Could you check a few things on this model? Use its own coordinates, in mm. Face numbers are marked on the shaded views. A direction names the side the tool comes from. Round coordinates to 2 decimals unless told otherwise and drop trailing zeros. Order: outer loops, then holes, each group sorted by start corner. A loop starts at its lowest first (then second) coordinate and runs counter-clockwise, first axis right, second up. Notation, with made-up numbers: (24.25, -19.5) -> (71.25, -19.5) arc R22 cw to (71.25, -9.5) -> close; hole circle Ø2 at (48, 9.25). An arc over 180 degrees is marked (long way). One line per question, with ' | ' between items.
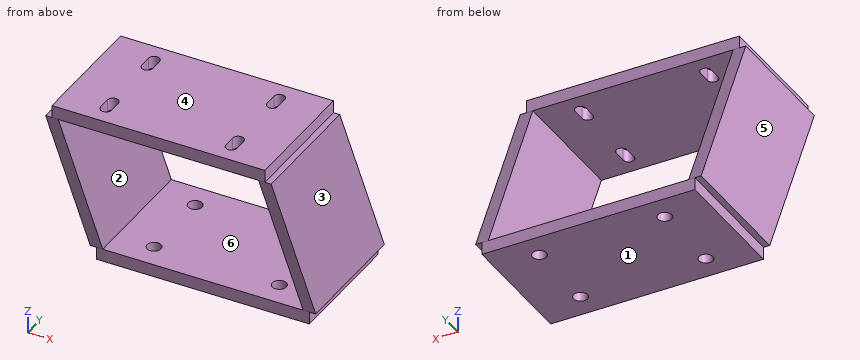
```python
from build123d import *

# Parameters (mm, degrees)
F0_W      = 215.9
F0_H      = 127
F1_DEPTH  = 12.7
F3_D      = 14.2875
F5_W      = 215.9
F5_H      = 127
F6_DEPTH  = 12.7
F8_DEPTH  = 212.726
F10_DEPTH = 6.35


# Not quite as in the source:
# - a length typed as a fraction of an inch, garbled in the dataset ("3 / 203.2 mm" for 3/8 in), is restored


with BuildPart() as f1:
    # F0 (on Top) → F1 (new body)
    with BuildSketch(Plane.XY):
        Rectangle(F0_W, F0_H)
    extrude(amount=F1_DEPTH)

    # F3 (through all)
    with Locations(Plane.XY.offset(12.7)):
        with Locations((-63.5, 38.1), (63.5, 38.1), (63.5, -38.1), (-63.5, -38.1)):
            Hole(F3_D / 2)



with BuildPart() as f6:
    # F5 (on offset) → F6 (new body)
    with BuildSketch(Plane.XY.offset(212.725)):
        with Locations((0, -82.55)):
            Rectangle(F5_W, F5_H)
    extrude(amount=-F6_DEPTH)

    # F7 (on face) → F8 (cut, through all)
    with BuildSketch(Plane.XY.offset(212.725)):
        with BuildLine():
            ThreePointArc((-57.94375, -38.1), (-63.5, -32.54375), (-69.05625, -38.1))
            Line((-69.05625, -38.1), (-69.05625, -50.8))
            ThreePointArc((-69.05625, -50.8), (-63.5, -56.35625), (-57.94375, -50.8))
            Line((-57.94375, -50.8), (-57.94375, -38.1))
        make_face()
        with BuildLine():
            ThreePointArc((-57.94375, -114.3), (-63.5, -108.74375), (-69.05625, -114.3))
            Line((-69.05625, -114.3), (-69.05625, -127))
            ThreePointArc((-69.05625, -127), (-63.5, -132.55625), (-57.94375, -127))
            Line((-57.94375, -127), (-57.94375, -114.3))
        make_face()
        with BuildLine():
            ThreePointArc((69.05625, -38.1), (63.5, -32.54375), (57.94375, -38.1))
            Line((57.94375, -38.1), (57.94375, -50.8))
            ThreePointArc((57.94375, -50.8), (63.5, -56.35625), (69.05625, -50.8))
            Line((69.05625, -50.8), (69.05625, -38.1))
        make_face()
        with BuildLine():
            ThreePointArc((69.05625, -114.3), (63.5, -108.74375), (57.94375, -114.3))
            Line((57.94375, -114.3), (57.94375, -127))
            ThreePointArc((57.94375, -127), (63.5, -132.55625), (69.05625, -127))
            Line((69.05625, -127), (69.05625, -114.3))
        make_face()
    extrude(amount=-F8_DEPTH, mode=Mode.SUBTRACT)


with BuildPart() as f1_1:
    add(f1.part)

    add(f6.part)  # F10 merges F6
    # F9 (on face) → F10 (join, symmetric)
    with BuildSketch(Plane.YZ.offset(107.95)):
        Polygon((63.5, 12.7), (-19.05, 200.025), (-146.05, 200.025), (-63.5, 12.7), align=None)
    extrude(amount=F10_DEPTH, both=True)

    # F11: F1 across plane


with BuildPart() as f1_2:
    add(f1_1.part)
    add(f1_1.part.mirror(Plane.YZ))


solid = f1_2.part
```
1. I want a section at A-A on x = 83. List the corners of the cut face in (y, z) for me (3 decimals), and give its area (3 significant figures).
From the geometry:
outline: (-146.05, 200.025) -> (-19.05, 200.025) -> (-19.05, 212.725) -> (-146.05, 212.725) -> close; (-63.5, 0) -> (63.5, 0) -> (63.5, 12.7) -> (-63.5, 12.7) -> close | area: 3,230 mm²
2. I want a section at D-D on y = -4.5. List the corners of the cut face in (x, z) for me, and give its area (3 significant figures).
From the geometry:
outline: (-114.3, 12.7) -> (-107.95, 12.7) -> (-107.95, 0) -> (107.95, 0) -> (107.95, 12.7) -> (114.3, 12.7) -> (114.3, 167.01) -> (101.6, 167.01) -> (101.6, 12.7) -> (-101.6, 12.7) -> (-101.6, 167.01) -> (-114.3, 167.01) -> close | area: 6,660 mm²
3. On a 3-axis mill with a long thin cutter (end or side, diameter ignored), from which of +Z, -Z, +X, -X, +Y, -Y can I reach the whole of each face in a straight line? I mean the marked faces 1 and 2. Say none if no direction works.
From the geometry:
face 1: -Z, +X, -X, +Y, -Y | face 2: +Y, -Y
4. I need wall thicknesses on probe 1 along X at (y, z) = (38, 9); probe 2 along Y at (x, z) = (-63.5, 9.75); probe 3 along X at (y, z) = (-40, 53). Which ranges of each line are inside material? Lowest first, please.
From the geometry:
probe 1: x = -107.95 to -70.64, -56.36 to 56.36, 70.64 to 107.95 | probe 2: y = -63.5 to -45.24, -30.96 to 30.96, 45.24 to 63.5 | probe 3: x = -114.3 to -101.6, 101.6 to 114.3
5. If we mould it in two halves opening along X, with no side actions, what happens to the marked faces 3, 4, 5 and 6? For each: pulls with the +X half, pulls with the -X half, needs draft (parallel to the pull), parting line crosses it, or undercut.
From the geometry:
face 3: pulls with the +X half | face 4: needs draft | face 5: pulls with the -X half | face 6: undercut
6. I want a section at B-B on z = 101. List the corners of the cut face in (x, y) for me.
From the geometry:
outline: (-114.3, -102.41) -> (-101.6, -102.41) -> (-101.6, 24.59) -> (-114.3, 24.59) -> close; (101.6, -102.41) -> (114.3, -102.41) -> (114.3, 24.59) -> (101.6, 24.59) -> close
7. I want a section at C-C on y = 38.1. List the corners of the cut face in (x, z) for me, and give its area (3 significant figures).
From the geometry:
outline: (-114.3, 12.7) -> (-107.95, 12.7) -> (-107.95, 0) -> (-70.64, 0) -> (-70.64, 12.7) -> (-101.6, 12.7) -> (-101.6, 70.34) -> (-114.3, 70.34) -> close; (-56.36, 0) -> (56.36, 0) -> (56.36, 12.7) -> (-56.36, 12.7) -> close; (70.64, 0) -> (107.95, 0) -> (107.95, 12.7) -> (114.3, 12.7) -> (114.3, 70.34) -> (101.6, 70.34) -> (101.6, 12.7) -> (70.64, 12.7) -> close | area: 3,840 mm²
8. I'm going to push flat-ended pins straight in: pin 1 (13 mm diameter, centred on x = 63.5, y = 38.1, fed in from +Z); pin 2 (14 mm diameter, centred on x = -51.5, z = 7, fed in from -Y); pin 3 (18.5 mm diameter, centred on x = -63.5, y = 38.1, fed in from +Z); pin 4 (1.9 mm diameter, centred on x = -110.5, y = -68, fed in from +Z) (3 decimals). Where does each tip first touch, or does it pass through?
From the geometry:
pin 1: passes through | pin 2: stops at y = -63.5 | pin 3: stops at z = 12.7 | pin 4: stops at z = 200.025
